Check sheet for the modelled part. Datum: model origin and axes. Units: mm. Face numbers are marked on the shaded views. Give positions to 0.01 mm unless a question says otherwise; leave off trailing zeros. Write each loop counter-clockwise with the first axis right and the second up, starting at its lowest first coordinate (ties: lowest second). Pieces come first, ordered by that corner, then holes.
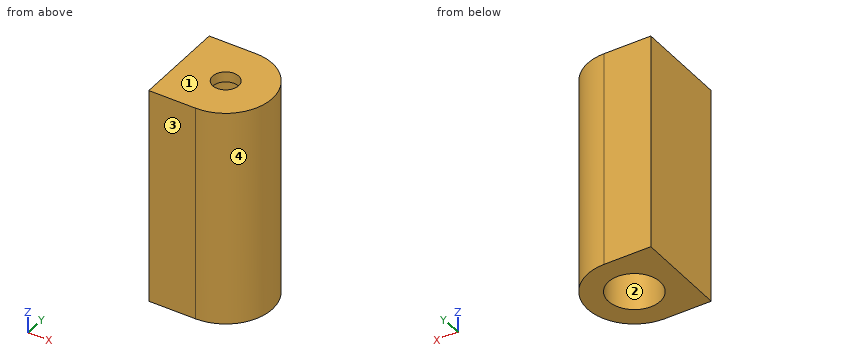
from build123d import *

# Parameters (mm, degrees)
F1_DEPTH = 40
F3_D     = 10
F3_DEPTH = 38.5
F3_TIP   = 3.0043030951
F4_DEPTH = 2


with BuildPart() as f1:
    # F0 (on Top) → F1 (new body)
    with BuildSketch(Plane.XY):
        with BuildLine():
            ThreePointArc((0, -5), (-5, 0), (0, 5))
            Line((0, 5), (0, 9))
            ThreePointArc((0, 9), (-6.3639610307, 6.3639610307), (-9, 0))
            ThreePointArc((-9, 0), (-6.3639610307, -6.3639610307), (0, -9))
            Line((0, -9), (0, -5))
        make_face()
        with BuildLine():
            ThreePointArc((-9, 0), (-6.3639610307, 6.3639610307), (0, 9))
            Line((0, 9), (-9, 9))
            Line((-9, 9), (-9, 0))
        make_face()
        with BuildLine():
            Line((-9, -9), (0, -9))
            ThreePointArc((0, -9), (-6.3639610307, -6.3639610307), (-9, 0))
            Line((-9, 0), (-9, -9))
        make_face()
        with BuildLine():
            ThreePointArc((0, 5), (3.5355339059, 3.5355339059), (5, 0))
            ThreePointArc((5, 0), (3.5355339059, -3.5355339059), (0, -5))
            Line((0, -5), (0, -9))
            ThreePointArc((0, -9), (6.3639610307, -6.3639610307), (9, 0))
            ThreePointArc((9, 0), (6.3639610307, 6.3639610307), (0, 9))
            Line((0, 9), (0, 5))
        make_face()
        with BuildLine():
            Line((0, -5), (0, 5))
            ThreePointArc((0, 5), (-5, 0), (0, -5))
        make_face()
        with BuildLine():
            ThreePointArc((0, -5), (3.5355339059, -3.5355339059), (5, 0))
            ThreePointArc((5, 0), (3.5355339059, 3.5355339059), (0, 5))
            Line((0, 5), (0, -5))
        make_face()
    extrude(amount=F1_DEPTH)

    # F3
    with Locations(Plane(origin=(0, 0, 0), x_dir=(1, 0, 0), z_dir=(0, 0, -1))):
        with Locations((0, 0)):
            Hole(F3_D / 2, depth=F3_DEPTH)
            with Locations((0, 0, -(F3_DEPTH + F3_TIP / 2))):  # 118° drill point
                Cone(0, F3_D / 2, F3_TIP, mode=Mode.SUBTRACT)

    # F4 (add): a face of the model
    f4_faces = [f1.faces().sort_by_distance(p)[0] for p in [
        (-4.5, 8.7454415588, 40),
    ]]
    extrude(f4_faces, amount=F4_DEPTH)


solid = f1.part
1) Scan lines: L1, parallel to Y at x = 0, z = 22; L2, parallel to Y at x = 0, z = 40.6; L3, parallel to X at y = 3.5, z = 20.5. Record each from-to range of solid material in increasing order.
2) Sectioned sample at B-B on z = 26. Record the boundary of the cut face in (x, y).
3) Sectioned sample at A-A on y = 0. Record the boundary of the cut face in (x, z).
4) Gauge pin test, flat ends, axial feed: pin 1 (1 mm diameter, centred on y = -4, z = 29, fed in from +X); pin 2 (3 mm diameter, centred on y = 2, z = 31, fed in from +X). Record the tip position at first contact, or that the pin passes through.
5) Sectioned sample at C-C on y = 5.5. Record the boundary of the cut face in (x, z), then the cut area to 3 significant figures.
6) Draft check along Y on the marked faces 1, 2, 3 and 4. Enter one of: +Y half, -Y half, draft (parallel to the pull), parting line (faces both ways), or undercut.
Answers below:
1. L1: y = -9 to -5, 5 to 9
1. L2: y = -9 to -2.5, 2.5 to 9
1. L3: x = -9 to -3.57, 3.57 to 8.29
2. outline: (-9, -9) - (0, -9) arc R9 ccw to (0, 9) - (-9, 9) - close; hole circle Ø10 at (0, 0)
3. outline: (-9, 0) - (-5, 0) - (-5, 38.5) - (-2.5, 40) - (-2.5, 42) - (-9, 42) - close; (2.5, 40) - (5, 38.5) - (5, 0) - (9, 0) - (9, 42) - (2.5, 42) - close
4. pin 1: stops at x = 8.29
4. pin 2: stops at x = 8.99
5. outline: (-9, 0) - (7.12, 0) - (7.12, 42) - (-9, 42) - close
5. area: 677 mm2
6. face 1: draft
6. face 2: undercut
6. face 3: -Y half
6. face 4: parting line
